Here's the drawing with two shaded views (mm, measured from the low corner). I have some questions. Give positions to 0.01 mm unless a question says otherwise; leave off trailing zeros.
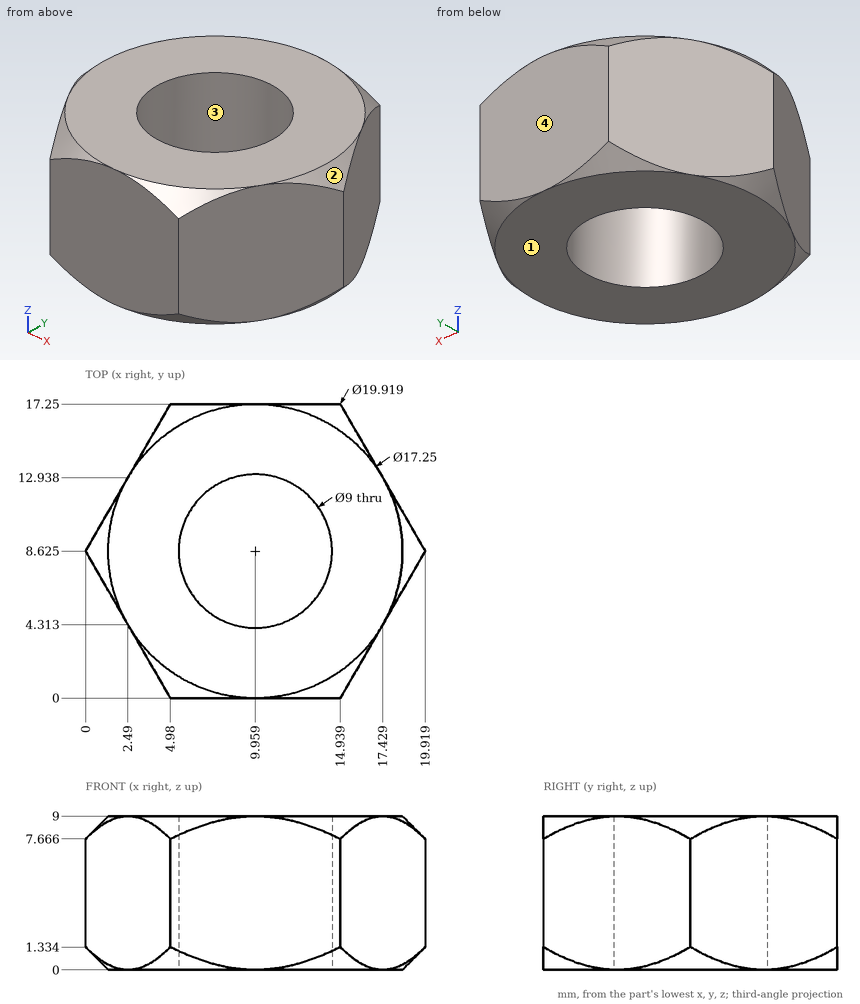
(1) Will these pins go through, and if not, where does the flat tip stop? P1, Ø4, axis at y = 8.5, z = 5, coming from the +X side; P2, Ø6, axis at x = 2, y = 11, coming from the -Z side; P3, Ø3, axis at y = 3.5, z = 5, coming from the -X side; P4, Ø2, axis at y = 2, z = 1.5, coming from the -X side.
Returned:
P1: stops at x = 19.92
P2: stops at z = 0
P3: stops at x = 2.09
P4: stops at x = 3.25
(2) If we mould it in two halves opening along Y, with no side actions, what happens to the marked faces 1, 2, 3 and 4? For each: +Y half, -Y half, draft (parallel to the pull), parting line (faces both ways), or undercut.
Returned:
face 1: draft
face 2: parting line
face 3: undercut
face 4: +Y half
(3) If I drill on L1, parallel to X at y = 9.5, z = 3.75 (1 decimal); L2, parallel to X at y = 6.25, z = 7.5 (1 decimal); L3, parallel to Y at x = 8.5, z = 6.25, over which ranges is the centre line in solid material (lowest first)?
Returned:
L1: x = 0.5 to 5.5, 14.4 to 19.4
L2: x = 1.4 to 6.1, 13.8 to 18.5
L3: y = 0 to 4.37, 12.88 to 17.25
